Design review of the part built by this model. Coordinates are the model's own, in mm. Face numbers are marked on the shaded views. A direction names the side the tool comes from. Give positions to 0.01 mm unless a question says otherwise; leave off trailing zeros. Order: outer loops, then holes, each group sorted by start corner. A loop starts at its lowest first (then second) coordinate and runs counter-clockwise, first axis right, second up. Notation, with made-up numbers: (-21.5, 0) -> (1.5, 0) arc R27 ccw to (1.5, 16) -> close; hole circle Ø9 at (56, -34). An arc over 180 degrees is marked (long way). One line per item, written item: value. Start each with the question number.
1) Wall thickness on line 1 along Y through (x, z) = (1.5, -13); line 2 along Z through (x, y) = (6.5, -1.55); line 3 along Y through (x, z) = (-0.5, -3.5): over which ranges is each line inside the solid? List them lowest first. Write a range as from..to.
2) Consider section A-A (y = -0.7). State the section outline as (x, z) points, plus the area to 3 significant figures.
3) For pin 1 (1 mm diameter, centred on y = -1.5, z = 11.5, fed in from +X); pin 2 (2.5 mm diameter, centred on y = -1, z = -17.5, fed in from +X); pin 3 (0.6 mm diameter, centred on y = -1, z = 16, fed in from -X), all flat-tipped, find the tip position at first contact; note any pin that passes through.
4) Consider section D-D (x = -1.5). State the section outline as (y, z) points.
5) The part is to be moulded in two halves that separate along X. For the marked faces 3 and 4, say which applies: released by +X, released by -X, zero draft, split by the parting line, or undercut.
6) Consider section B-B (x = 7). State the section outline as (y, z) points.
7) Tool access review of the marked faces 1 and 2: name each direction out of +Z, -Z, +X, -X, +Y, -Y from which nothing blocks a thin tool from reaching the whole face with its end or side.
8) Consider section C-C (z = -3). State the section outline as (x, y) points (3 decimals), plus the area to 3 significant figures.
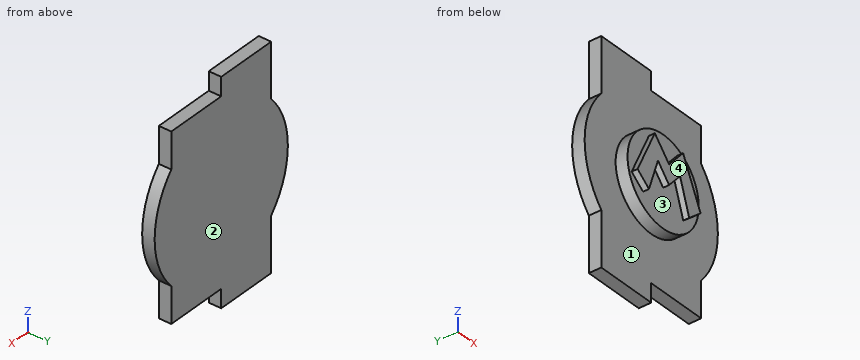
from build123d import *

# Parameters (mm, degrees)
F1_DEPTH = 2.1
F3_DEPTH = 3
F2_R     = 7.4807460639
F4_DEPTH = 2


# Not quite as in the source:
# - a feature names something its author has since deleted; it is built from what else it names


with BuildPart() as f1:
    # F0 (on Front) → F1 (new body)
    with BuildSketch(Plane.XZ):
        with BuildLine():
            Line((0, 15.3), (0, 18.4))
            Line((0, 18.4), (-10.5, 18.4))
            Line((-10.5, 18.4), (-10.5, 9.2601295887))
            ThreePointArc((-10.5, 9.2601295887), (-14, 0), (-10.5, -9.2601295887))
            Line((-10.5, -9.2601295887), (-10.5, -18.4))
            Line((-10.5, -18.4), (0, -18.4))
            Line((0, -18.4), (0, -15.3))
            Line((0, -15.3), (10.5, -15.3))
            Line((10.5, -15.3), (10.5, -9.2601295887))
            ThreePointArc((10.5, -9.2601295887), (14, 0), (10.5, 9.2601295887))
            Line((10.5, 9.2601295887), (10.5, 15.3))
            Line((10.5, 15.3), (0, 15.3))
        make_face()
    extrude(amount=F1_DEPTH)

    # F2 (on face) → F3 (join)
    with BuildSketch(Plane.XZ.offset(2.1)):
        Polygon((-2.9942439869, 5.6681009009), (-6.6190003417, -1.9491401035), (-4.228762351, -3.8665838074), (-2.3375852033, 1.6756160185), (0, -0.9772852063), (2.3115586955, 1.6493498115), (4.2290021665, -3.9453827776), (6.6192396916, -1.9491401035), (2.9419509228, 5.6681009009), (0, 2.3060084786), align=None)
    extrude(amount=F3_DEPTH)

    # F2 (on face) → F4 (join)
    with BuildSketch(Plane.XZ.offset(2.1)):
        Circle(F2_R)
        Polygon((-4.228762351, -3.8665838074), (-6.6190003417, -1.9491401035), (-2.9942439869, 5.6681009009), (0, 2.3060084786), (2.9419509228, 5.6681009009), (6.6192396916, -1.9491401035), (4.2290021665, -3.9453827776), (2.3115586955, 1.6493498115), (0, -0.9772852063), (-2.3375852033, 1.6756160185), align=None, mode=Mode.SUBTRACT)
    extrude(amount=F4_DEPTH)


solid = f1.part
Checked values:
1. line 1: y = -2.1..0
1. line 2: z = -15.3..15.3
1. line 3: y = -4.1..0
2. outline: (-10.5, -18.4) -> (0, -18.4) -> (0, -15.3) -> (10.5, -15.3) -> (10.5, -9.26) arc R14 ccw to (10.5, 9.26) -> (10.5, 15.3) -> (0, 15.3) -> (0, 18.4) -> (-10.5, 18.4) -> (-10.5, 9.26) arc R14 ccw to (-10.5, -9.26) -> close
2. area: 797 mm^2
3. pin 1: stops at x = 10.5
3. pin 2: stops at x = 0
3. pin 3: stops at x = -10.5
4. outline: (-5.1, 0.73) -> (-4.1, 0.73) -> (-4.1, -7.33) -> (-2.1, -7.33) -> (-2.1, -18.4) -> (0, -18.4) -> (0, 18.4) -> (-2.1, 18.4) -> (-2.1, 7.33) -> (-4.1, 7.33) -> (-4.1, 3.99) -> (-5.1, 3.99) -> close
5. face 3: undercut
5. face 4: zero draft
6. outline: (-4.1, -2.64) -> (-2.1, -2.64) -> (-2.1, -15.3) -> (0, -15.3) -> (0, 15.3) -> (-2.1, 15.3) -> (-2.1, 2.64) -> (-4.1, 2.64) -> close
7. face 1: -Y
7. face 2: +Z, -Z, +X, -X, +Y
8. outline: (-13.675, -2.1) -> (-6.853, -2.1) -> (-6.853, -4.1) -> (-5.309, -4.1) -> (-5.309, -5.1) -> (-3.933, -5.1) -> (-3.933, -4.1) -> (3.905, -4.1) -> (3.905, -5.1) -> (5.361, -5.1) -> (5.361, -4.1) -> (6.853, -4.1) -> (6.853, -2.1) -> (13.675, -2.1) -> (13.675, 0) -> (-13.675, 0) -> close
8. area: 87.7 mm^2
